The listing builds one solid part. Answer for the finished solid, in the listing's coordinates (mm). A direction names the side the tool comes from. Coordinates: 2 decimals unless noted, no trailing zeros. Order: outer loops, then holes, each group sorted by start corner. A loop starts at its lowest first (then second) coordinate and runs counter-clockwise, first axis right, second up. Notation, with made-up numbers: (-32.5, 39.25) - (-8.5, 39.25) arc R22 cw to (-8.5, 63.25) - close; hole circle Ø3 at (-38.5, 9.25). An arc over 180 degrees is marked (long way). Use a Markdown table: item, result. Add a question column.
Item 1: The mould has two halves that part along Y. Classify faces 5 (the cylindrical face through (-11.99, 34.897, 13.465)), 6 (the cylindrical face through (-2.19, 20.85, 13.54)), 7 (the flat face through (17, 8, 11)): released by +Y, released by -Y, zero draft, split by the parting line, or undercut.
Item 2: Find the intervals of material crossed by line 1 along Z through (x, y) = (8, -43); line 2 along Z through (x, y) = (6.5, 5.5); line 3 along Y through (x, z) = (4.5, 17.45), in increasing order.
Item 3: The part is cut by section A-A, the plane y = -32. Give the vertices of the cut face in (x, z), then the cut area to 3 significant figures.
Item 4: The part is cut by section B-B, the plane z = -8. Give the vertices of the cut face in (x, y), then the cut area to 3 significant figures.
Item 5: The part is cut by section C-C, the plane x = 10.5. State how many separate pieces and enclosed holes the cut face has, then the cut area to 3 significant figures.
Item 6: The part is cut by section D-D, the plane y = 16. Give the vertices of the cut face in (x, z), then the cut area to 3 significant figures.
Item 7: Flat-ended cylindrical pins translate along their axes: P1, Ø1, axis at x = 2, y = 0.5, coming from the +Z side; P2, Ø6, axis at x = 21.2, y = 9, coming from the -Z side; P3, Ø3.5, axis at x = 4.5, y = -46, coming from the +Z side (1 decimal); P4, Ø18.5, axis at x = 15.5, y = 13.5, coming from the +Z side. Find the tip coordinate at first contact, or state that the pin passes through.
Item 8: For faces 1 (the flat face through (13, 18, 14)), 2 (the flat face through (4.8, 8, 0)), 3 (the flat face through (4, 11, -16)), 4 (the cylindrical face through (4.86, -4.86, -15.1)), determine the directions among +Z, -Z, +X, -X, +Y, -Y from which every point of the face is accessible in a straight line to the end or side of a thin tool.
from build123d import *

# Parameters (mm, degrees)
SKETCH1_R              = 2.5
SKETCH1_R_2            = 2.25
BOSS_EXTRUDE1_DEPTH    = 16
CUT_EXTRUDE_START      = -27
CUT_EXTRUDE_4_DEPTH    = 27
EXTRUDE_1_DEPTH        = 55
EXTRUDE_1_DEPTH_BACK   = 5
SKETCH_8_W             = 51.4
SKETCH_8_H             = 5
EXTRUDE_1_2_DEPTH      = 55
EXTRUDE_1_2_DEPTH_BACK = 5
FILLET_1_R             = 3
FILLET_2_R             = 3
FILLET_3_R             = 3
FILLET_4_R             = 3
SKETCH_9_W             = 25.4
SKETCH_9_H             = 19.916079783
CUT_EXTRUDE_5_DEPTH    = 11
SKETCH_10_R            = 2
CUT_EXTRUDE_6_DEPTH    = 79.466808437


with BuildPart() as part:
    # Sketch1 → Boss-Extrude1 (new, symmetric)
    with BuildSketch(Plane.XY):
        with BuildLine():
            Line((-21.2, 33), (-21.2, 22))
            Line((-21.2, 22), (-21.2, 0))
            Line((-21.2, 0), (-21.2, -4))
            Line((-21.2, -4), (30.2, -4))
            Line((30.2, -4), (30.2, 9))
            ThreePointArc((30.2, 9), (27.563961031, 15.363961031), (21.2, 18))
            Line((21.2, 18), (4.8, 18))
            ThreePointArc((4.8, 18), (-2.271067812, 20.928932188), (-5.2, 28))
            Line((-5.2, 28), (-5.2, 33))
            ThreePointArc((-5.2, 33), (-13.2, 41), (-21.2, 33))
        make_face()
        with Locations((21.2, 9)):
            Circle(SKETCH1_R, mode=Mode.SUBTRACT)
        with Locations((-13.2, 33)):
            Circle(SKETCH1_R_2, mode=Mode.SUBTRACT)
    extrude(amount=BOSS_EXTRUDE1_DEPTH, both=True)

    # 草图7 → 切除-拉伸4 (cut)
    with BuildSketch(Plane(origin=(0, 0, -16), x_dir=(-1, 0, 0), z_dir=(0, 0, -1)).offset(CUT_EXTRUDE_START)):
        with BuildLine():
            Line((-4.8, 18), (21.2, 18))
            Line((21.2, 18), (21.2, 33))
            ThreePointArc((21.2, 33), (13.2, 41), (5.2, 33))
            Line((5.2, 33), (5.2, 28))
            ThreePointArc((5.2, 28), (2.271067812, 20.928932188), (-4.8, 18))
        make_face()
    extrude(amount=CUT_EXTRUDE_4_DEPTH, mode=Mode.SUBTRACT)


with BuildPart() as body_2:
    # 草图8 → 凸台-拉伸1 (new, two sides: drawn at the far end of the back side and taken through both)
    with BuildSketch(Plane.XZ.offset(4).offset(-EXTRUDE_1_DEPTH_BACK)):
        with Locations((4.5, 18.5)):
            Rectangle(SKETCH_8_W, SKETCH_8_H)
    extrude(amount=EXTRUDE_1_DEPTH + EXTRUDE_1_DEPTH_BACK)


with BuildPart() as body_3:
    # 草图8 → Extrude 1 2 (new, two sides: drawn at the far end of the back side and taken through both)
    with BuildSketch(Plane.XZ.offset(4).offset(-EXTRUDE_1_2_DEPTH_BACK)):
        with Locations((4.5, -18.5)):
            Rectangle(SKETCH_8_W, SKETCH_8_H)
    extrude(amount=EXTRUDE_1_2_DEPTH + EXTRUDE_1_2_DEPTH_BACK)

    # Combine 1: union part, body 2
    add(part.part)
    add(body_2.part)

    # 圆角1
    fillet_1_edges = [body_3.edges().sort_by_distance(p)[0] for p in [
        (4.5, 1, -16),
    ]]
    fillet(fillet_1_edges, radius=FILLET_1_R)

    # 圆角2
    fillet_2_edges = [body_3.edges().sort_by_distance(p)[0] for p in [
        (4.5, 1, 16),
    ]]
    fillet(fillet_2_edges, radius=FILLET_2_R)

    # 圆角3
    fillet_3_edges = [body_3.edges().sort_by_distance(p)[0] for p in [
        (4.5, -4, -16),
        (4.5, -4, 16),
    ]]
    fillet(fillet_3_edges, radius=FILLET_3_R)

    # 圆角4
    fillet_4_edges = [body_3.edges().sort_by_distance(p)[0] for p in [
        (4.5, 1, 21),
        (4.5, 1, -21),
    ]]
    fillet(fillet_4_edges, radius=FILLET_4_R)

    # 草图9 → 切除-拉伸5 (cut, symmetric)
    with BuildSketch(Plane.XY):
        with Locations((17.5, 8.041960108)):
            Rectangle(SKETCH_9_W, SKETCH_9_H)
    extrude(amount=CUT_EXTRUDE_5_DEPTH, both=True, mode=Mode.SUBTRACT)

    # 草图10 → 切除-拉伸6 (cut, through all)
    with BuildSketch(Plane(origin=(0, 0, -21), x_dir=(-1, 0, 0), z_dir=(0, 0, -1))):
        with Locations((2.5, -39)):
            Circle(SKETCH_10_R)
        with Locations((-4.5, -32)):
            Circle(SKETCH_10_R)
        with Locations((-4.5, -46)):
            Circle(SKETCH_10_R)
        with Locations((-11.5, -39)):
            Circle(SKETCH_10_R)
    extrude(amount=-CUT_EXTRUDE_6_DEPTH, mode=Mode.SUBTRACT)


solid = body_3.part
Solution:
| question | item | result |
|---|---|---|
| 1 | face 5 | undercut |
| 1 | face 6 | released by +Y |
| 1 | face 7 | zero draft |
| 2 | line 1 | z = -21 to -16, 16 to 21 |
| 2 | line 2 | z = -16 to -11, 11 to 16 |
| 2 | line 3 | y = -59 to -48, -44 to -34, -30 to 1.43 |
| 3 | outline | (-21.2, -21) - (2.5, -21) - (2.5, -16) - (-21.2, -16) - close; (-21.2, 16) - (2.5, 16) - (2.5, 21) - (-21.2, 21) - close; (6.5, -21) - (30.2, -21) - (30.2, -16) - (6.5, -16) - close; (6.5, 16) - (30.2, 16) - (30.2, 21) - (6.5, 21) - close |
| 3 | area | 474 mm2 |
| 4 | outline | (-21.2, -4) - (30.2, -4) - (30.2, -1.92) - (4.8, -1.92) - (4.8, 18) - (-21.2, 18) - close |
| 4 | area | 625 mm2 |
| 5 | separate pieces | 3 |
| 5 | enclosed holes | 0 |
| 5 | area | 835 mm2 |
| 6 | outline | (-21.2, -16) - (26.86, -16) - (26.86, -11) - (4.8, -11) - (4.8, 11) - (26.86, 11) - (26.86, 16) - (-21.2, 16) - close |
| 6 | area | 1,050 mm2 |
| 7 | P1 | stops at z = 20.31 |
| 7 | P2 | stops at z = -16 |
| 7 | P3 | passes through |
| 7 | P4 | stops at z = 16 |
| 8 | face 1 | +Z, -Z, +X, +Y |
| 8 | face 2 | +X, +Y |
| 8 | face 3 | -Z, +X, -X, +Y |
| 8 | face 4 | +X, -X, -Y |
